Can you work these out from the model? Positions are in its coordinate system, mm. Face numbers are marked on the shaded views. A direction names the side the tool comes from. Give positions to 0.01 mm unless a question says otherwise; leave off trailing zeros. Order: outer loops, then holes, each group sorted by start corner. A loop starts at its lowest first (then second) coordinate and runs counter-clockwise, first axis right, second up.
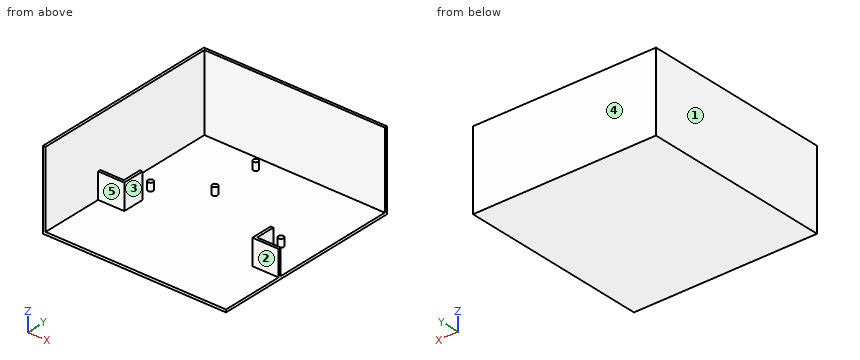
```python
from build123d import *

# Parameters (mm, degrees)
F0_W     = 105
F0_H     = 110
F1_DEPTH = 1.5
F2_W     = 105
F2_H     = 1.5
F3_DEPTH = 43.5
F4_W     = 1.5
F4_H     = 108.5
F5_DEPTH = 43.5
F6_R     = 1.5
F7_DEPTH = 4.5
F8_W     = 1.5
F8_H     = 11
F9_DEPTH = 14.6


with BuildPart() as f1:
    # F0 (on Top) → F1 (new body)
    with BuildSketch(Plane.XY):
        Rectangle(F0_W, F0_H)
    extrude(amount=F1_DEPTH)

    # F2 (on face) → F3 (join)
    with BuildSketch(Plane.XY.offset(1.5)):
        with Locations((0, 54.25)):
            Rectangle(F2_W, F2_H)
    extrude(amount=F3_DEPTH)

    # F4 (on face) → F5 (join)
    with BuildSketch(Plane.XY.offset(1.5)):
        with Locations((-51.75, -0.75)):
            Rectangle(F4_W, F4_H)
    extrude(amount=F5_DEPTH)

    # F6 (on face) → F7 (join)
    with BuildSketch(Plane.XY.offset(1.5)):
        with Locations((-14.8, 45.5)):
            Circle(F6_R)
        with Locations((-14.8, 17.56)):
            Circle(F6_R)
        with Locations((-38.9, 2.3)):
            Circle(F6_R)
        with Locations((36, 2.3)):
            Circle(F6_R)
    extrude(amount=F7_DEPTH)

    # F8 (on face) → F9 (join)
    with BuildSketch(Plane.XY.offset(1.5)):
        Polygon((-37.5, -17.6), (-51, -17.6), (-51, -19.1), (-36, -19.1), (-36, -17.6), align=None)
        with Locations((-36.75, -12.1)):
            Rectangle(F8_W, F8_H)
        Polygon((37.5, -19.1), (52.5, -19.1), (52.5, -17.6), (39, -17.6), (37.5, -17.6), align=None)
        with Locations((38.25, -12.1)):
            Rectangle(F8_W, F8_H)
    extrude(amount=F9_DEPTH)


solid = f1.part
```
1) Suppose I cut it at C-C (y = 2.3). Please give me the cut outline in (x, z).
2) I'm going to push flat-ended pins straight in: pin 1 Ø8 at (y, z) = (-33, 7.5) entering from +X; pin 2 Ø1.5 at (x, y) = (36.5, 2) entering from +Z; pin 3 Ø12 at (x, z) = (17.5, 15.5) entering from -Y. Where does each tip first touch, or does it pass through?
3) Suppose I cut it at B-B (x = -38.9). Please give me the cut outline in (y, z), and give its area (3 significant figures).
4) Which directions (+Z, -Z, +X, -X, +Y, -Y) give clear straight access to the entire face, cutting with the end or side of a thin tool? Please do the marked faces 4 and 5.
5) Suppose I cut it at D-D (z = 31). Please give me the cut outline in (x, y), and give its area (3 significant figures).
6) If I drill on line 1 (Y direction, x = 43, z = 4); line 2 (Y direction, x = -33, z = 7.5); line 3 (X direction, y = 27, z = 35), over which ranges is the centre line in solid material (lowest first)?
7) We'd pull the mould along X, two halves only. Please class the marked faces 1, 2 and 3: +X half, -X half, draft (parallel to the pull), parting line (faces both ways), or undercut.
8) Suppose I cut it at A-A (z = 14). Please give me the cut outline in (x, y).
Results:
1. outline: (-52.5, 0) - (52.5, 0) - (52.5, 1.5) - (37.5, 1.5) - (37.5, 6) - (34.5, 6) - (34.5, 1.5) - (-37.4, 1.5) - (-37.4, 6) - (-40.4, 6) - (-40.4, 1.5) - (-51, 1.5) - (-51, 45) - (-52.5, 45) - close
2. pin 1: stops at x = -51
2. pin 2: stops at z = 6
2. pin 3: stops at y = 53.5
3. outline: (-55, 0) - (55, 0) - (55, 45) - (53.5, 45) - (53.5, 1.5) - (3.8, 1.5) - (3.8, 6) - (0.8, 6) - (0.8, 1.5) - (-17.6, 1.5) - (-17.6, 16.1) - (-19.1, 16.1) - (-19.1, 1.5) - (-55, 1.5) - close
3. area: 266 mm2
4. face 4: +Z, -Z, +X, -X, +Y
4. face 5: +Z, +X, -Y
5. outline: (-52.5, -55) - (-51, -55) - (-51, 53.5) - (52.5, 53.5) - (52.5, 55) - (-52.5, 55) - close
5. area: 320 mm2
6. line 1: y = -19.1 to -17.6, 53.5 to 55
6. line 2: y = 53.5 to 55
6. line 3: x = -52.5 to -51
7. face 1: -X half
7. face 2: draft
7. face 3: undercut
8. outline: (-52.5, -55) - (-51, -55) - (-51, -19.1) - (-36, -19.1) - (-36, -6.6) - (-37.5, -6.6) - (-37.5, -17.6) - (-51, -17.6) - (-51, 53.5) - (52.5, 53.5) - (52.5, 55) - (-52.5, 55) - close; (37.5, -19.1) - (52.5, -19.1) - (52.5, -17.6) - (39, -17.6) - (39, -6.6) - (37.5, -6.6) - close
